Part model, mm, in its own coordinate system. A direction names the side the tool comes from. Coordinates: 2 decimals unless noted, no trailing zeros.
1) Pin check, flat tips, straight feed: pin 1 Ø1 at (x, z) = (-2, 3.5) entering from -Y; pin 2 Ø1 at (x, y) = (-2.5, 1.5) entering from +Z; pin 3 Ø3 at (y, z) = (-3, 14) entering from -X. Stop position of each tip, or through.
2) Wall check: L1, parallel to Z at x = -2.75, y = 1; L2, parallel to Y at x = 0, z = 6.25; L3, parallel to X at y = 0.5, z = 8.75. Give the ranges that are in metal, low to high.
3) Tool access for faces 1 (the cylindrical face through (1.27, -2.44, 14.15)), 2 (the cylindrical face through (-0.613, -3.517, 6.902)), 3 (the cylindrical face through (-0.627, 3.515, 6.902)): list every direction of +Z, -Z, +X, -X, +Y, -Y with a clear straight run to the whole face (end or side of a thin tool).
4) Mould opens along Y. For faces 4 (the cylindrical face through (2.54, -1.05, -0.15)), 5 (the cylindrical face through (3.36, -1.21, 6.9)), 6 (the cylindrical face through (1.79, -3.09, 6.9)), 7 (the cylindrical face through (3.35, 1.23, 6.9)) say: +Y half, -Y half, draft (parallel to the pull), parting line (faces both ways), or undercut.
```python
from build123d import *

# Parameters (mm, degrees)
SKETCH2_R           = 2
BOSS_EXTRUDE1_DEPTH = 14
SKETCH3_R           = 2.75
BOSS_EXTRUDE2_DEPTH = 14.5
SKETCH4_R           = 2.75
BOSS_EXTRUDE3_DEPTH = 0.5
SKETCH5_R           = 1.995
BOSS_EXTRUDE4_DEPTH = 2
SKETCH6_R           = 1.995
BOSS_EXTRUDE5_DEPTH = 2
SKETCH7_R           = 0.6
CUT_EXTRUDE1_DEPTH  = 21
CHAMFER1_SIZE       = 0.2


with BuildPart() as part:
    # Sketch2 → Boss-Extrude1 (new body)
    with BuildSketch(Plane.XY):
        with BuildLine():
            Line((-4.409637173, -1.2), (-3.764514138, -0.899174188))
            ThreePointArc((-3.764514138, -0.899174188), (-3.582420347, -0.728223333), (-3.537232834, -0.482580436))
            ThreePointArc((-3.537232834, -0.482580436), (-3.57, 0), (-3.537232834, 0.482580436))
            ThreePointArc((-3.537232834, 0.482580436), (-3.582420347, 0.728223333), (-3.764514138, 0.899174188))
            Line((-3.764514138, 0.899174188), (-4.409637173, 1.2))
            ThreePointArc((-4.409637173, 1.2), (-4.294395277, 1.563032055), (-4.149323184, 1.915206806))
            Line((-4.149323184, 1.915206806), (-3.461763164, 1.730975654))
            ThreePointArc((-3.461763164, 1.730975654), (-3.212386135, 1.744883974), (-3.019874282, 1.904011377))
            ThreePointArc((-3.019874282, 1.904011377), (-2.734778662, 2.294751767), (-2.399480831, 2.6433675))
            ThreePointArc((-2.399480831, 2.6433675), (-2.276200264, 2.860586849), (-2.305807109, 3.108590435))
            Line((-2.305807109, 3.108590435), (-2.606632921, 3.75371347))
            ThreePointArc((-2.606632921, 3.75371347), (-2.285, 3.957736095), (-1.947494763, 4.134267063))
            Line((-1.947494763, 4.134267063), (-1.539214732, 3.55118275))
            ThreePointArc((-1.539214732, 3.55118275), (-1.339240749, 3.401540677), (-1.089482991, 3.399695106))
            ThreePointArc((-1.089482991, 3.399695106), (-0.619923994, 3.515763678), (-0.13898508, 3.567293533))
            ThreePointArc((-0.13898508, 3.567293533), (0.095079219, 3.654449987), (0.231812692, 3.863462669))
            Line((0.231812692, 3.863462669), (0.416043844, 4.551022689))
            ThreePointArc((0.416043844, 4.551022689), (0.793572172, 4.500571431), (1.165588102, 4.418857814))
            Line((1.165588102, 4.418857814), (1.10354938, 3.709751971))
            ThreePointArc((1.10354938, 3.709751971), (1.160550267, 3.466578694), (1.3506895, 3.304623712))
            ThreePointArc((1.3506895, 3.304623712), (1.785, 3.091710692), (2.186543334, 2.822043275))
            ThreePointArc((2.186543334, 2.822043275), (2.421870079, 2.738355361), (2.660964759, 2.810577782))
            Line((2.660964759, 2.810577782), (3.244049071, 3.218857814))
            ThreePointArc((3.244049071, 3.218857814), (3.500823105, 2.937539376), (3.73327934, 2.635815883))
            Line((3.73327934, 2.635815883), (3.229950472, 2.132487015))
            ThreePointArc((3.229950472, 2.132487015), (3.117306916, 1.909566013), (3.158859362, 1.663282156))
            ThreePointArc((3.158859362, 1.663282156), (3.354702656, 1.221011912), (3.488963822, 0.756327606))
            ThreePointArc((3.488963822, 0.756327606), (3.615441013, 0.540953828), (3.845021841, 0.442592316))
            Line((3.845021841, 0.442592316), (4.554127684, 0.380553593))
            ThreePointArc((4.554127684, 0.380553593), (4.57, 0), (4.554127684, -0.380553593))
            Line((4.554127684, -0.380553593), (3.845021841, -0.442592316))
            ThreePointArc((3.845021841, -0.442592316), (3.615441013, -0.540953828), (3.488963822, -0.756327606))
            ThreePointArc((3.488963822, -0.756327606), (3.354702656, -1.221011912), (3.158859362, -1.663282156))
            ThreePointArc((3.158859362, -1.663282156), (3.117306916, -1.909566013), (3.229950472, -2.132487015))
            Line((3.229950472, -2.132487015), (3.73327934, -2.635815883))
            ThreePointArc((3.73327934, -2.635815883), (3.500823105, -2.937539376), (3.244049071, -3.218857814))
            Line((3.244049071, -3.218857814), (2.660964759, -2.810577782))
            ThreePointArc((2.660964759, -2.810577782), (2.421870079, -2.738355361), (2.186543334, -2.822043275))
            ThreePointArc((2.186543334, -2.822043275), (1.785, -3.091710692), (1.3506895, -3.304623712))
            ThreePointArc((1.3506895, -3.304623712), (1.160550267, -3.466578694), (1.10354938, -3.709751971))
            Line((1.10354938, -3.709751971), (1.165588102, -4.418857814))
            ThreePointArc((1.165588102, -4.418857814), (0.793572172, -4.500571431), (0.416043844, -4.551022689))
            Line((0.416043844, -4.551022689), (0.231812692, -3.863462669))
            ThreePointArc((0.231812692, -3.863462669), (0.095079219, -3.654449987), (-0.13898508, -3.567293533))
            ThreePointArc((-0.13898508, -3.567293533), (-0.619923994, -3.515763678), (-1.089482991, -3.399695106))
            ThreePointArc((-1.089482991, -3.399695106), (-1.339240749, -3.401540677), (-1.539214732, -3.55118275))
            Line((-1.539214732, -3.55118275), (-1.947494763, -4.134267063))
            ThreePointArc((-1.947494763, -4.134267063), (-2.285, -3.957736095), (-2.606632921, -3.75371347))
            Line((-2.606632921, -3.75371347), (-2.305807109, -3.108590435))
            ThreePointArc((-2.305807109, -3.108590435), (-2.276200264, -2.860586849), (-2.399480831, -2.6433675))
            ThreePointArc((-2.399480831, -2.6433675), (-2.734778662, -2.294751767), (-3.019874282, -1.904011377))
            ThreePointArc((-3.019874282, -1.904011377), (-3.212386135, -1.744883974), (-3.461763164, -1.730975654))
            Line((-3.461763164, -1.730975654), (-4.149323184, -1.915206806))
            ThreePointArc((-4.149323184, -1.915206806), (-4.294395277, -1.563032055), (-4.409637173, -1.2))
        make_face()
        Circle(SKETCH2_R, mode=Mode.SUBTRACT)
    extrude(amount=BOSS_EXTRUDE1_DEPTH)

    # Sketch3 → Boss-Extrude2 (add)
    with BuildSketch(Plane.XY.offset(14)):
        Circle(SKETCH3_R)
    extrude(amount=-BOSS_EXTRUDE2_DEPTH)

    # Sketch4 → Boss-Extrude3 (add)
    with BuildSketch(Plane.XY.offset(14)):
        Circle(SKETCH4_R)
    extrude(amount=BOSS_EXTRUDE3_DEPTH)

    # Sketch5 → Boss-Extrude4 (add)
    with BuildSketch(Plane.XY.offset(14.5)):
        Circle(SKETCH5_R)
    extrude(amount=BOSS_EXTRUDE4_DEPTH)

    # Sketch6 → Boss-Extrude5 (add)
    with BuildSketch(Plane(origin=(0, 0, -0.5), x_dir=(-1, 0, 0), z_dir=(0, 0, -1))):
        Circle(SKETCH6_R)
    extrude(amount=BOSS_EXTRUDE5_DEPTH)

    # Sketch7 → Cut-Extrude1 (cut)
    with BuildSketch(Plane(origin=(0, 0, -2.5), x_dir=(-1, 0, 0), z_dir=(0, 0, -1))):
        Circle(SKETCH7_R)
    extrude(amount=-CUT_EXTRUDE1_DEPTH, mode=Mode.SUBTRACT)

    # Chamfer1
    chamfer1_edges = [part.edges().sort_by_distance(p)[0] for p in [
        (-2.75, 0, -0.5),
        (-2.75, 0, 14.5),
        (-1.995, 0, 16.5),
        (1.995, 0, -2.5),
    ]]
    chamfer(chamfer1_edges, length=CHAMFER1_SIZE)


solid = part.part
```
Geometry check:
1. pin 1: stops at y = -4.13
1. pin 2: stops at z = 14.5
1. pin 3: stops at x = -4.32
2. L1: z = 0 to 14
2. L2: y = -3.6 to -0.6, 0.6 to 3.6
2. L3: x = -3.54 to -0.33, 0.33 to 3.67
3. face 1: +Z
3. face 2: +Z, -Z, -Y
3. face 3: +Z, -Z, +Y
4. face 4: parting line
4. face 5: undercut
4. face 6: -Y half
4. face 7: undercut
